```python
from build123d import *

# Parameters (mm, degrees)
SKETCH1_R             = 45
SKETCH1_R_2           = 1.5
BOSS_EXTRUDE2_DEPTH   = 5
SKETCH9_R             = 3.937
BOSS_EXTRUDE7_DEPTH   = 4
SKETCH10_R            = 1.7
CUT_EXTRUDE9_DEPTH    = 14
M3_TAPPED_HOLE1_D     = 2.5
M3_TAPPED_HOLE1_DEPTH = 7
M3_TAPPED_HOLE1_TIP   = 0.751075774


with BuildPart() as part:
    # Sketch1 → Boss-Extrude2 (new body)
    with BuildSketch(Plane(origin=(0, 0, 0), x_dir=(1, 0, 0), z_dir=(0, 1, 0))):
        with Locations(Location((0, 0, 0), (0, 0, 270))):
            Circle(SKETCH1_R)
        with Locations(Location((0, 41.75, 0), (0, 0, 270))):
            Circle(SKETCH1_R_2, mode=Mode.SUBTRACT)
        with Locations(Location((29.521708115, 29.521708115, 0), (0, 0, 270))):
            Circle(SKETCH1_R_2, mode=Mode.SUBTRACT)
        with Locations(Location((41.75, 0, 0), (0, 0, 270))):
            Circle(SKETCH1_R_2, mode=Mode.SUBTRACT)
        with Locations(Location((29.521708115, -29.521708115, 0), (0, 0, 270))):
            Circle(SKETCH1_R_2, mode=Mode.SUBTRACT)
        with Locations(Location((0, -41.75, 0), (0, 0, 270))):
            Circle(SKETCH1_R_2, mode=Mode.SUBTRACT)
        with Locations(Location((-29.521708115, -29.521708115, 0), (0, 0, 270))):
            Circle(SKETCH1_R_2, mode=Mode.SUBTRACT)
        with Locations(Location((-41.75, 0, 0), (0, 0, 270))):
            Circle(SKETCH1_R_2, mode=Mode.SUBTRACT)
        with Locations(Location((-29.521708115, 29.521708115, 0), (0, 0, 270))):
            Circle(SKETCH1_R_2, mode=Mode.SUBTRACT)
    extrude(amount=BOSS_EXTRUDE2_DEPTH)

    # Sketch9 → Boss-Extrude7 (add)
    with BuildSketch(Plane.XZ):
        with Locations(Location((27, 0, 0), (0, 0, 90))):
            Circle(SKETCH9_R)
        with Locations(Location((0, -27, 0), (0, 0, 90))):
            Circle(SKETCH9_R)
        with Locations(Location((-27, 0, 0), (0, 0, 90))):
            Circle(SKETCH9_R)
        with Locations(Location((0, 27, 0), (0, 0, 90))):
            Circle(SKETCH9_R)
    extrude(amount=BOSS_EXTRUDE7_DEPTH)

    # Sketch10 → Cut-Extrude9 (cut)
    with BuildSketch(Plane(origin=(0, 5, 0), x_dir=(1, 0, 0), z_dir=(0, 1, 0))):
        with Locations(Location((0, 41.75, 0), (0, 0, 270))):
            Circle(SKETCH10_R)
        with Locations(Location((29.521708115, 29.521708115, 0), (0, 0, 270))):
            Circle(SKETCH10_R)
        with Locations(Location((41.75, 0, 0), (0, 0, 270))):
            Circle(SKETCH10_R)
        with Locations(Location((29.521708115, -29.521708115, 0), (0, 0, 270))):
            Circle(SKETCH10_R)
        with Locations(Location((0, -41.75, 0), (0, 0, 270))):
            Circle(SKETCH10_R)
        with Locations(Location((-29.521708115, -29.521708115, 0), (0, 0, 270))):
            Circle(SKETCH10_R)
        with Locations(Location((-41.75, 0, 0), (0, 0, 270))):
            Circle(SKETCH10_R)
        with Locations(Location((-29.521708115, 29.521708115, 0), (0, 0, 270))):
            Circle(SKETCH10_R)
    extrude(amount=-CUT_EXTRUDE9_DEPTH, mode=Mode.SUBTRACT)

    # M3 Tapped Hole1
    with Locations(Plane.XZ.offset(4)):
        with Locations((0, 27), (27, 0), (0, -27), (-27, 0)):
            Hole(M3_TAPPED_HOLE1_D / 2, depth=M3_TAPPED_HOLE1_DEPTH)
            with Locations((0, 0, -(M3_TAPPED_HOLE1_DEPTH + M3_TAPPED_HOLE1_TIP / 2))):  # 118° drill point
                Cone(0, M3_TAPPED_HOLE1_D / 2, M3_TAPPED_HOLE1_TIP, mode=Mode.SUBTRACT)


solid = part.part
```
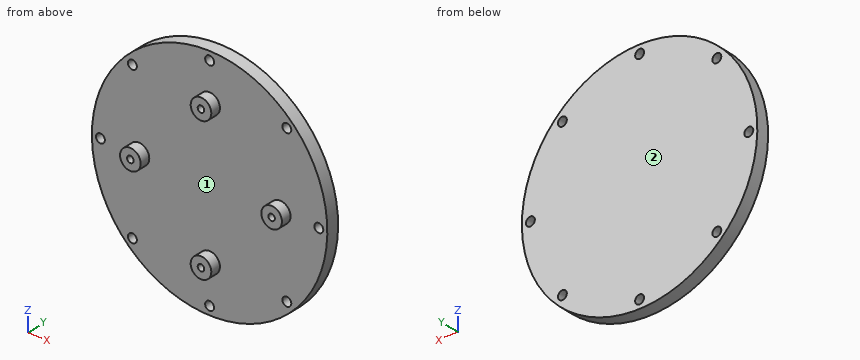
The listing builds one solid part. Answer for the finished solid, in the listing's coordinates (mm). Face numbers are marked on the shaded views. A direction names the side the tool comes from. Round coordinates to 2 decimals unless told otherwise and drop trailing zeros. Order: outer loops, then holes, each group sorted by start corner. A loop starts at its lowest first (then second) coordinate and runs counter-clockwise, first axis right, second up. Notation, with made-up numbers: (8.5, 85) -> (12.5, 85) arc R22 ccw to (12.5, 98) -> close; hole circle Ø4 at (-5.75, 71.25). An arc over 180 degrees is marked (long way). Answer as CSV lines item,"result".
Q1. A cutting plane is placed at A-A on y = -2. Determine the outline of the cut face in (x, z), plus the area to 3 significant figures.
Computed values:
outline,"circle Ø7.87 at (-27, 0); circle Ø7.87 at (0, -27); circle Ø7.87 at (0, 27); circle Ø7.87 at (27, 0); hole circle Ø2.5 at (-27, 0); hole circle Ø2.5 at (0, -27); hole circle Ø2.5 at (0, 27); hole circle Ø2.5 at (27, 0)"
area,"175 mm^2"
Q2. Which of the six approach directions +Z, -Z, +X, -X, +Y, -Y give full straight-line access (tool end or side, diameter ignored) to the marked faces 1 and 2?
Computed values:
face 1,"-Y"
face 2,"+Z, -Z, +X, -X, +Y"
Q3. Given pin 1 (4.5 mm diameter, centred on x = -29.52, z = -29.52, fed in from -Y); pin 2 (5.5 mm diameter, centred on x = 0, z = -41.75, fed in from +Y); pin 3 (3 mm diameter, centred on x = 0, z = 41.75, fed in from -Y); pin 4 (4 mm diameter, centred on x = 4.5, y = -1.5, fed in from +Z), each flat-ended and moving along its own axis, determine where each tip first touches the part or whether it passes through.
Computed values:
pin 1,"stops at y = 0"
pin 2,"stops at y = 5"
pin 3,"passes through"
pin 4,"stops at z = 44.89"
Q4. A cutting plane is placed at B-B on x = -41.75. Determine the outline of the cut face in (y, z).
Computed values:
outline,"(0, -16.79) -> (5, -16.79) -> (5, -1.7) -> (0, -1.7) -> close; (0, 1.7) -> (5, 1.7) -> (5, 16.79) -> (0, 16.79) -> close"
Q5. A cutting plane is placed at C-C on z = 41.75. Determine the outline of the cut face in (x, y).
Computed values:
outline,"(-16.79, 0) -> (-1.7, 0) -> (-1.7, 5) -> (-16.79, 5) -> close; (1.7, 0) -> (16.79, 0) -> (16.79, 5) -> (1.7, 5) -> close"
Q6. Consider line 1 (X direction, y = 1.45, z = 0); line 2 (X direction, y = -1.25, z = 0); line 3 (X direction, y = 4, z = -30). Determine where each line is inside the solid, lowest interval first. Write a range as from..to.
Computed values:
line 1,"x = -45..-43.45, -40.05..-28.25, -25.75..25.75, 28.25..40.05, 43.45..45"
line 2,"x = -30.94..-28.25, -25.75..-23.06, 23.06..25.75, 28.25..30.94"
line 3,"x = -33.54..-31.15, -27.89..27.89, 31.15..33.54"
